```python
from build123d import *

# Parameters (mm, degrees)
EXTRUDE_1_DEPTH            = 65
SKETCH_2_R                 = 3
EXTRUDE_2_DEPTH            = 4
CHAMFER_1_SIZE             = 1
CHAMFER_1_OF_MIRROR_1_SIZE = 1


with BuildPart() as part:
    # 草圖1 → 伸長1 (new, symmetric)
    with BuildSketch(Plane.XY):
        with BuildLine():
            Line((-5, 20), (-5, -20))
            ThreePointArc((-5, -20), (0, -25), (5, -20))
            Line((5, -20), (5, 20))
            ThreePointArc((5, 20), (0, 25), (-5, 20))
        make_face()
    extrude(amount=EXTRUDE_1_DEPTH, both=True)

    # 草圖2 → 伸長2 (add)
    with BuildSketch(Plane.XY.offset(65)):
        with Locations(Location((0, 9.5, 0), (0, 0, 180))):
            Circle(SKETCH_2_R)
        with Locations(Location((0, -9.5, 0), (0, 0, 180))):
            Circle(SKETCH_2_R)
    extrude_2 = extrude(amount=EXTRUDE_2_DEPTH)

    # 導角1
    chamfer_1_edges = [part.edges().sort_by_distance(p)[0] for p in [
        (3, 9.5, 69),
        (3, -9.5, 69),
    ]]
    chamfer(chamfer_1_edges, length=CHAMFER_1_SIZE)

    # 鏡射1: 伸長2 across plane
    add(extrude_2.mirror(Plane.XY))

    # 導角1 of 鏡射1
    chamfer_1_of_mirror_1_edges = [part.edges().sort_by_distance(p)[0] for p in [
        (3, 9.5, -69),
        (3, -9.5, -69),
    ]]
    chamfer(chamfer_1_of_mirror_1_edges, length=CHAMFER_1_OF_MIRROR_1_SIZE)


solid = part.part
```
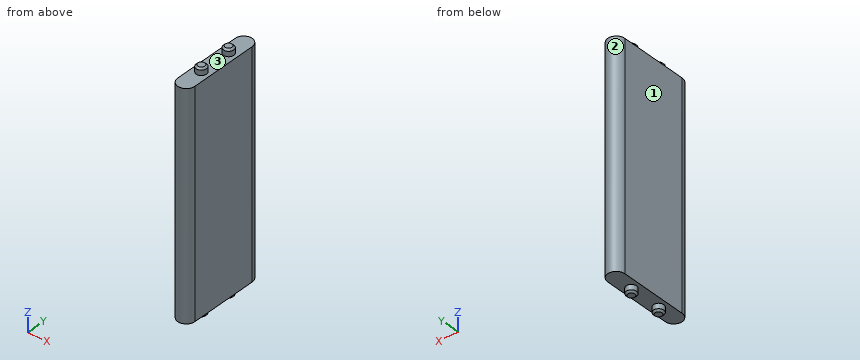
CAD build for the part. Positions are in the model's coordinates, mm. Face numbers are marked on the shaded views. Give positions to 0.01 mm unless a question says otherwise; leave off trailing zeros. Loops run counter-clockwise (first coordinate to the right, second up) from the corner with the lowest first, then second, coordinate; pieces in that order, holes last. Notation, with made-up numbers: (49, 63) -> (65, 63) arc R24 ccw to (65, 94) -> close; hole circle Ø5 at (-10.75, 30.25). An arc over 180 degrees is marked (long way). Use a Markdown table: item, result.
1. Slice it at D-D (y = 14). List the corners of the cut face in (x, z), plus the area to 3 significant figures.
Check result:
| item | result |
|---|---|
| outline | (-5, -65) -> (5, -65) -> (5, 65) -> (-5, 65) -> close |
| area | 1,300 mm^2 |
2. Mould opens along Y. For the marked faces 1, 2 and 3 say: pulls with the +Y half, pulls with the -Y half, needs draft (parallel to the pull), parting line crosses it, or undercut.
Check result:
| item | result |
|---|---|
| face 1 | needs draft |
| face 2 | pulls with the +Y half |
| face 3 | undercut |
3. Wall check: L1, parallel to Z at x = -0.25, y = -1; L2, parallel to Y at x = 0.5, z = 19.5; L3, parallel to Y at x = -3, z = 33. Give the ranges that are in metal, low to high. Write a range as [from, to].
Check result:
| item | result |
|---|---|
| L1 | z = [-65, 65] |
| L2 | y = [-24.97, 24.97] |
| L3 | y = [-24, 24] |
4. Flat gauge pins, fed straight in: pin 1 (3 mm diameter, centred on x = 1, y = -5, fed in from +Z); pin 2 (5 mm diameter, centred on x = 4, y = -2.5, fed in from -Z); pin 3 (1 mm diameter, centred on x = -2.5, z = -25.5, fed in from -Y). Where does each tip first touch, or does it go through?
Check result:
| item | result |
|---|---|
| pin 1 | stops at z = 65 |
| pin 2 | stops at z = -65 |
| pin 3 | stops at y = -24.58 |
5. Slice it at B-B (y = -9.5). List the corners of the cut face in (x, z).
Check result:
| item | result |
|---|---|
| outline | (-5, -65) -> (-3, -65) -> (-3, -68) -> (-2, -69) -> (2, -69) -> (3, -68) -> (3, -65) -> (5, -65) -> (5, 65) -> (3, 65) -> (3, 68) -> (2, 69) -> (-2, 69) -> (-3, 68) -> (-3, 65) -> (-5, 65) -> close |
6. Slice it at C-C (z = -9). List the corners of the cut face in (x, y).
Check result:
| item | result |
|---|---|
| outline | (-5, -20) arc R5 ccw to (5, -20) -> (5, 20) arc R5 ccw to (-5, 20) -> close |
7. Slice it at A-A (x = 0). List the corners of the cut face in (y, z), plus the area to 3 significant figures.
Check result:
| item | result |
|---|---|
| outline | (-25, -65) -> (-12.5, -65) -> (-12.5, -68) -> (-11.5, -69) -> (-7.5, -69) -> (-6.5, -68) -> (-6.5, -65) -> (6.5, -65) -> (6.5, -68) -> (7.5, -69) -> (11.5, -69) -> (12.5, -68) -> (12.5, -65) -> (25, -65) -> (25, 65) -> (12.5, 65) -> (12.5, 68) -> (11.5, 69) -> (7.5, 69) -> (6.5, 68) -> (6.5, 65) -> (-6.5, 65) -> (-6.5, 68) -> (-7.5, 69) -> (-11.5, 69) -> (-12.5, 68) -> (-12.5, 65) -> (-25, 65) -> close |
| area | 6,590 mm^2 |
